Part model, mm, in its own coordinate system. Face numbers are marked on the shaded views. Coordinates: 2 decimals unless noted, no trailing zeros. Loops run counter-clockwise (first coordinate to the right, second up) from the corner with the lowest first, then second, coordinate; pieces in that order, holes last. Notation, with made-up numbers: (-25.75, 9.25) - (16.25, 9.25) arc R13 ccw to (16.25, 19.25) - close; hole circle Ø1 at (69.25, 38). An arc over 180 degrees is marked (long way). One line per question, with ' | ' between items. Start each with the question number.
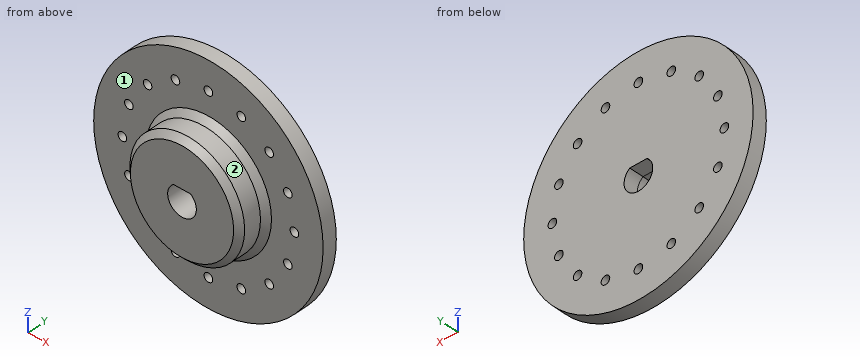
from build123d import *

# Parameters (mm, degrees)
F0_R     = 40
F0_R_2   = 1.5
F1_DEPTH = 5
F2_R     = 20
F3_DEPTH = 10
F4_DEPTH = 5.001
F5_SIZE  = 2


with BuildPart() as f1:
    # F0 (on Front) → F1 (new body)
    with BuildSketch(Plane.XZ):
        Circle(F0_R)
        with Locations((-21.213203, -21.213203)):
            Circle(F0_R_2, mode=Mode.SUBTRACT)
        with Locations((-11.480503, -27.716386)):
            Circle(F0_R_2, mode=Mode.SUBTRACT)
        with Locations((-27.716386, -11.480503)):
            Circle(F0_R_2, mode=Mode.SUBTRACT)
        with Locations((0, -30)):
            Circle(F0_R_2, mode=Mode.SUBTRACT)
        with Locations((11.480503, -27.716386)):
            Circle(F0_R_2, mode=Mode.SUBTRACT)
        with Locations((21.213203, -21.213203)):
            Circle(F0_R_2, mode=Mode.SUBTRACT)
        with Locations((27.716386, -11.480503)):
            Circle(F0_R_2, mode=Mode.SUBTRACT)
        with Locations((-30, 0)):
            Circle(F0_R_2, mode=Mode.SUBTRACT)
        with Locations((-27.716386, 11.480503)):
            Circle(F0_R_2, mode=Mode.SUBTRACT)
        with Locations((-21.213203, 21.213203)):
            Circle(F0_R_2, mode=Mode.SUBTRACT)
        with Locations((-11.480503, 27.716386)):
            Circle(F0_R_2, mode=Mode.SUBTRACT)
        with Locations((30, 0)):
            Circle(F0_R_2, mode=Mode.SUBTRACT)
        with Locations((27.716386, 11.480503)):
            Circle(F0_R_2, mode=Mode.SUBTRACT)
        with Locations((11.480503, 27.716386)):
            Circle(F0_R_2, mode=Mode.SUBTRACT)
        with Locations((0, 30)):
            Circle(F0_R_2, mode=Mode.SUBTRACT)
        with Locations((21.213203, 21.213203)):
            Circle(F0_R_2, mode=Mode.SUBTRACT)
    extrude(amount=F1_DEPTH)

    # F2 (on face) → F3 (join)
    with BuildSketch(Plane.XZ.offset(5)):
        Circle(F2_R)
        with BuildLine():
            ThreePointArc((3, 4), (0, -5), (-3, 4))
            Line((-3, 4), (3, 4))
        make_face(mode=Mode.SUBTRACT)
    extrude(amount=F3_DEPTH)

    # F3_face (on face) → F4 (cut, through all)
    with BuildSketch(Plane(origin=(0, -5, -0.241766), x_dir=(1, 0, 0), z_dir=(0, -1, 0))):
        with BuildLine():
            ThreePointArc((-3, 4.241766), (0, -4.758234), (3, 4.241766))
            Line((3, 4.241766), (-3, 4.241766))
        make_face()
    extrude(amount=-F4_DEPTH, mode=Mode.SUBTRACT)

    # F5
    f5_edges = [f1.edges().sort_by_distance(p)[0] for p in [
        (-20, -15, 0),
        (-20, -5, 0),
    ]]
    chamfer(f5_edges, length=F5_SIZE)


solid = f1.part
1) Band-saw the part on A-A on x = 0. List the corners of the cut face in (y, z), then the cut area to 3 significant figures.
2) Mould opens along Z. For the marked faces 1 and 2 say: +Z half, -Z half, draft (parallel to the pull), parting line (faces both ways), or undercut.
3) Band-saw the part on C-C on y = -2. Count the separate pieces of the cut face and the enclosed holes in it, then the cut area to 3 significant figures.
4) Band-saw the part on D-D on y = -6. List the corners of the cut face in (x, z).
5) Pin check, flat tips, straight feed: pin 1 Ø4 at (y, z) = (-6.5, 6.5) entering from -X; pin 2 Ø4 at (x, y) = (-14, -8.5) entering from -Z; pin 3 Ø2.5 at (x, z) = (0, -30) entering from +Y; pin 4 Ø6 at (x, z) = (-21, 28.5) entering from -Y. Stop position of each tip, or through.
6) Band-saw the part on B-B on y = -11.75. List the corners of the cut face in (x, z).
7) Wall check: line 1 along Z through (x, y) = (0, -1.8); line 2 along X through (y, z) = (-3.25, -22); line 3 along Y through (x, z) = (-15.5, -31). Give the ranges that are in metal, low to high. Write a range as [from, to].
Values found:
1) outline: (-15, -18) - (-13, -20) - (-7, -20) - (-5, -22) - (-5, -28.5) - (0, -28.5) - (0, -5) - (-15, -5) - close; (-15, 4) - (0, 4) - (0, 28.5) - (-5, 28.5) - (-5, 22) - (-7, 20) - (-13, 20) - (-15, 18) - close; (-5, -40) - (0, -40) - (0, -31.5) - (-5, -31.5) - close; (-5, 31.5) - (0, 31.5) - (0, 40) - (-5, 40) - close | area: 635 mm²
2) face 1: draft | face 2: parting line
3) separate pieces: 1 | enclosed holes: 17 | area: 4,840 mm²
4) outline: circle Ø42 at (0, 0); hole (-3, 4) arc R5 ccw (long way) to (3, 4) - close
5) pin 1: x = -39.66 | pin 2: z = -16 | pin 3: through | pin 4: y = -5
6) outline: circle Ø40 at (0, 0); hole (-3, 4) arc R5 ccw (long way) to (3, 4) - close
7) line 1: [-40, -31.5], [-28.5, -5], [4, 28.5], [31.5, 40] | line 2: [-33.41, -22.49], [-19.94, 19.94], [22.49, 33.41] | line 3: [-5, 0]
